CAD build for the part. Positions are in the model's coordinates, mm. Face numbers are marked on the shaded views. A direction names the side the tool comes from. Give positions to 0.01 mm unless a question says otherwise; leave off trailing zeros. Write each loop counter-clockwise with the first axis right and the second up, starting at its lowest first coordinate (ties: lowest second). Pieces come first, ordered by that corner, then holes. Notation, with made-up numbers: (-19.75, -39.75) - (12.25, -39.75) arc R22 cw to (12.25, -13.75) - close; hole circle Ø2 at (-32.75, 2). An arc over 180 degrees is marked (long way). Answer as a JSON object with one key per item and string values.
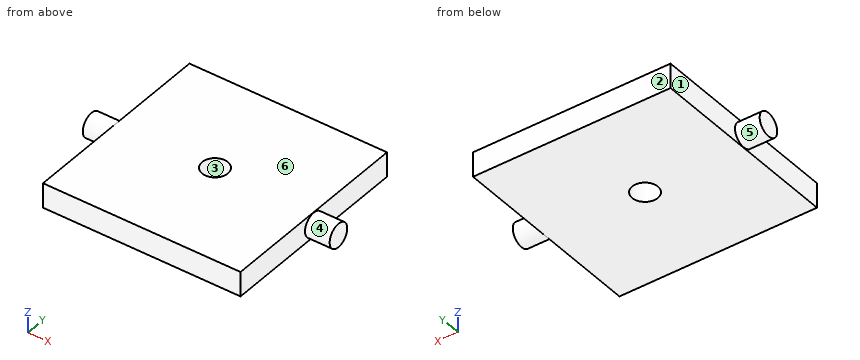
from build123d import *

# Parameters (mm, degrees)
F0_W     = 40
F0_H     = 40
F1_DEPTH = 5
F2_R     = 2.6
F3_DEPTH = 25.4
F4_R     = 2.4
F5_DEPTH = 5


with BuildPart() as f1:
    # F0 (on Top) → F1 (new body)
    with BuildSketch(Plane.XY):
        Rectangle(F0_W, F0_H)
    extrude(amount=F1_DEPTH)

    # F2 (on face) → F3 (cut)
    with BuildSketch(Plane.XY.offset(5)):
        Circle(F2_R)
    extrude(amount=-F3_DEPTH, mode=Mode.SUBTRACT)

    # F4 (on face) → F5 (join)
    with BuildSketch(Plane.YZ.offset(20)):
        with Locations((0, 2.5)):
            Circle(F4_R)
    extrude(amount=F5_DEPTH)

    # F6: F1 across plane


with BuildPart() as f1_1:
    add(f1.part)
    add(f1.part.mirror(Plane.YZ))


solid = f1_1.part
(1) 3-axis set-ups, long thin cutter, end or side, ignore diameter. For the marked faces 4, 5 and 6: which of +Z, -Z, +X, -X, +Y, -Y reach the whole face in a straight line?
Answer key:
{"face 4": "+X", "face 5": "-X", "face 6": "+Z, +X, -X, +Y, -Y"}
(2) Saw through at C-C, the plane z = 1.8. Give the cut face in (x, y).
Answer key:
{"outline": "(-25, -2.3) - (-20, -2.3) - (-20, -20) - (20, -20) - (20, -2.3) - (25, -2.3) - (25, 2.3) - (20, 2.3) - (20, 20) - (-20, 20) - (-20, 2.3) - (-25, 2.3) - close; hole circle Ø5.2 at (0, 0)"}
(3) Saw through at D-D, the plane y = -15.5. Give the cut face in (x, z), and give its area (3 significant figures).
Answer key:
{"outline": "(-20, 0) - (20, 0) - (20, 5) - (-20, 5) - close", "area": "200 mm²"}
(4) Saw through at A-A, the plane y = 0. Give the cut face in (x, z).
Answer key:
{"outline": "(-25, 0.1) - (-20, 0.1) - (-20, 0) - (-2.6, 0) - (-2.6, 5) - (-20, 5) - (-20, 4.9) - (-25, 4.9) - close; (2.6, 0) - (20, 0) - (20, 0.1) - (25, 0.1) - (25, 4.9) - (20, 4.9) - (20, 5) - (2.6, 5) - close"}
(5) Probe L1, parallel to X at y = 0, z = 4; L2, parallel to Y at x = 0, z = 2.5; L3, parallel to X at y = -3, z = 1.8. List the from-to ranges inside material, lowest first. Write a range as [from, to].
Answer key:
{"L1": "x = [-25, -2.6], [2.6, 25]", "L2": "y = [-20, -2.6], [2.6, 20]", "L3": "x = [-20, 20]"}
(6) Flat gauge pin, fed straight in: P1, Ø1, axis at y = 10.5, z = 4, coming from the -X side. Where does the tip first touch, or does it go through?
Answer key:
{"P1": "stops at x = -20"}
(7) Saw through at B-B, the plane x = 0. Give the cut face in (y, z), and give its area (3 significant figures).
Answer key:
{"outline": "(-20, 0) - (-2.6, 0) - (-2.6, 5) - (-20, 5) - close; (2.6, 0) - (20, 0) - (20, 5) - (2.6, 5) - close", "area": "174 mm²"}
(8) Pull direction Y, two halves, no side cores. Call the marked faces 1, 2 and 3: pulls with the +Y half, pulls with the -Y half, needs draft (parallel to the pull), parting line crosses it, or undercut.
Answer key:
{"face 1": "needs draft", "face 2": "pulls with the +Y half", "face 3": "undercut"}
